Geometry: final body of the model. Coordinates: model frame, mm. Give positions to 0.01 mm unless a question says otherwise; leave off trailing zeros. Use a Markdown table: item, result. Add a question column.
1) Line query: line 1 (Z direction, x = 44, y = 15); line 2 (Z direction, x = 335.5, y = -21.5); line 3 (Z direction, x = -232.5, y = 0.5). Output: solid intervals per line, ascending.
2) Pin query (flat end, axial travel): pin 1 (1.9 mm diameter, centred on x = 117, z = -14.5, fed in from +Y). Return the tip coordinate at first contact, or that it passes through.
3) Section A-A on x = -64.5. State how many separate pieces and enclosed holes the cut face has, then the cut area to 3 significant figures.
```python
from build123d import *

# Parameters (mm, degrees)
SKETCH_14_R                 = 3
SKETCH_14_R_2               = 2.5
GB_T5237_2004_6060G_1_DEPTH = 850


with BuildPart() as part:
    # 草图14 → 铝型材（gb t5237-2004） 6060G(1) (new body)
    with BuildSketch(Plane.YZ.offset(-425)):
        with BuildLine():
            Line((28, -18.15), (30, -18.15))
            Line((30, -18.15), (30, -29.5))
            ThreePointArc((30, -29.5), (29.853553391, -29.853553391), (29.5, -30))
            Line((29.5, -30), (18.15, -30))
            Line((18.15, -30), (18.15, -28))
            Line((18.15, -28), (20.15, -28))
            Line((20.15, -28), (20.15, -22))
            Line((20.15, -22), (18.15, -22))
            Line((18.15, -22), (18.15, -20))
            Line((18.15, -20), (11.85, -20))
            Line((11.85, -20), (11.85, -22))
            Line((11.85, -22), (9.85, -22))
            Line((9.85, -22), (9.85, -28))
            Line((9.85, -28), (11.85, -28))
            Line((11.85, -28), (11.85, -30))
            Line((11.85, -30), (-11.85, -30))
            Line((-11.85, -30), (-11.85, -28))
            Line((-11.85, -28), (-9.85, -28))
            Line((-9.85, -28), (-9.85, -22))
            Line((-9.85, -22), (-11.85, -22))
            Line((-11.85, -22), (-11.85, -20))
            Line((-11.85, -20), (-18.15, -20))
            Line((-18.15, -20), (-18.15, -22))
            Line((-18.15, -22), (-20.15, -22))
            Line((-20.15, -22), (-20.15, -28))
            Line((-20.15, -28), (-18.15, -28))
            Line((-18.15, -28), (-18.15, -30))
            Line((-18.15, -30), (-29.5, -30))
            ThreePointArc((-29.5, -30), (-29.853553391, -29.853553391), (-30, -29.5))
            Line((-30, -29.5), (-30, -18.15))
            Line((-30, -18.15), (-28, -18.15))
            Line((-28, -18.15), (-28, -20.15))
            Line((-28, -20.15), (-22, -20.15))
            Line((-22, -20.15), (-22, -18.15))
            Line((-22, -18.15), (-20, -18.15))
            Line((-20, -18.15), (-20, -11.85))
            Line((-20, -11.85), (-22, -11.85))
            Line((-22, -11.85), (-22, -9.85))
            Line((-22, -9.85), (-28, -9.85))
            Line((-28, -9.85), (-28, -11.85))
            Line((-28, -11.85), (-30, -11.85))
            Line((-30, -11.85), (-30, 11.85))
            Line((-30, 11.85), (-28, 11.85))
            Line((-28, 11.85), (-28, 9.85))
            Line((-28, 9.85), (-22, 9.85))
            Line((-22, 9.85), (-22, 11.85))
            Line((-22, 11.85), (-20, 11.85))
            Line((-20, 11.85), (-20, 18.15))
            Line((-20, 18.15), (-22, 18.15))
            Line((-22, 18.15), (-22, 20.15))
            Line((-22, 20.15), (-28, 20.15))
            Line((-28, 20.15), (-28, 18.15))
            Line((-28, 18.15), (-30, 18.15))
            Line((-30, 18.15), (-30, 29.5))
            ThreePointArc((-30, 29.5), (-29.853553391, 29.853553391), (-29.5, 30))
            Line((-29.5, 30), (-18.15, 30))
            Line((-18.15, 30), (-18.15, 28))
            Line((-18.15, 28), (-20.15, 28))
            Line((-20.15, 28), (-20.15, 22))
            Line((-20.15, 22), (-18.15, 22))
            Line((-18.15, 22), (-18.15, 20))
            Line((-18.15, 20), (-11.85, 20))
            Line((-11.85, 20), (-11.85, 22))
            Line((-11.85, 22), (-9.85, 22))
            Line((-9.85, 22), (-9.85, 28))
            Line((-9.85, 28), (-11.85, 28))
            Line((-11.85, 28), (-11.85, 30))
            Line((-11.85, 30), (11.85, 30))
            Line((11.85, 30), (11.85, 28))
            Line((11.85, 28), (9.85, 28))
            Line((9.85, 28), (9.85, 22))
            Line((9.85, 22), (11.85, 22))
            Line((11.85, 22), (11.85, 20))
            Line((11.85, 20), (18.15, 20))
            Line((18.15, 20), (18.15, 22))
            Line((18.15, 22), (20.15, 22))
            Line((20.15, 22), (20.15, 28))
            Line((20.15, 28), (18.15, 28))
            Line((18.15, 28), (18.15, 30))
            Line((18.15, 30), (29.5, 30))
            ThreePointArc((29.5, 30), (29.853553391, 29.853553391), (30, 29.5))
            Line((30, 29.5), (30, 18.15))
            Line((30, 18.15), (28, 18.15))
            Line((28, 18.15), (28, 20.15))
            Line((28, 20.15), (22, 20.15))
            Line((22, 20.15), (22, 18.15))
            Line((22, 18.15), (20, 18.15))
            Line((20, 18.15), (20, 11.85))
            Line((20, 11.85), (22, 11.85))
            Line((22, 11.85), (22, 9.85))
            Line((22, 9.85), (28, 9.85))
            Line((28, 9.85), (28, 11.85))
            Line((28, 11.85), (30, 11.85))
            Line((30, 11.85), (30, -11.85))
            Line((30, -11.85), (28, -11.85))
            Line((28, -11.85), (28, -9.85))
            Line((28, -9.85), (22, -9.85))
            Line((22, -9.85), (22, -11.85))
            Line((22, -11.85), (20, -11.85))
            Line((20, -11.85), (20, -18.15))
            Line((20, -18.15), (22, -18.15))
            Line((22, -18.15), (22, -20.15))
            Line((22, -20.15), (28, -20.15))
            Line((28, -20.15), (28, -18.15))
        make_face()
        with Locations((25, 25)):
            Circle(SKETCH_14_R, mode=Mode.SUBTRACT)
        with Locations((-15, 15)):
            Circle(SKETCH_14_R_2, mode=Mode.SUBTRACT)
        with Locations((-25, -25)):
            Circle(SKETCH_14_R, mode=Mode.SUBTRACT)
        with Locations((25, -25)):
            Circle(SKETCH_14_R, mode=Mode.SUBTRACT)
        with Locations((15, -15)):
            Circle(SKETCH_14_R_2, mode=Mode.SUBTRACT)
        with Locations((-15, -15)):
            Circle(SKETCH_14_R_2, mode=Mode.SUBTRACT)
        with Locations((-25, 25)):
            Circle(SKETCH_14_R, mode=Mode.SUBTRACT)
        with Locations((15, 15)):
            Circle(SKETCH_14_R_2, mode=Mode.SUBTRACT)
        with BuildLine():
            Line((18.15, -10.5), (20.8, -7.85))
            Line((20.8, -7.85), (22.5, -7.85))
            ThreePointArc((22.5, -7.85), (25.328427125, -6.678427125), (26.5, -3.85))
            Line((26.5, -3.85), (26.5, 3.85))
            ThreePointArc((26.5, 3.85), (25.328427125, 6.678427125), (22.5, 7.85))
            Line((22.5, 7.85), (20.8, 7.85))
            Line((20.8, 7.85), (18.15, 10.5))
            Line((18.15, 10.5), (15, 10.5))
            ThreePointArc((15, 10.5), (11.818019485, 11.818019485), (10.5, 15))
            Line((10.5, 15), (10.5, 18.15))
            Line((10.5, 18.15), (7.85, 20.8))
            Line((7.85, 20.8), (7.85, 22.5))
            ThreePointArc((7.85, 22.5), (6.678427125, 25.328427125), (3.85, 26.5))
            Line((3.85, 26.5), (-3.85, 26.5))
            ThreePointArc((-3.85, 26.5), (-6.678427125, 25.328427125), (-7.85, 22.5))
            Line((-7.85, 22.5), (-7.85, 20.8))
            Line((-7.85, 20.8), (-10.5, 18.15))
            Line((-10.5, 18.15), (-10.5, 15))
            ThreePointArc((-10.5, 15), (-11.818019485, 11.818019485), (-15, 10.5))
            Line((-15, 10.5), (-18.15, 10.5))
            Line((-18.15, 10.5), (-20.8, 7.85))
            Line((-20.8, 7.85), (-22.5, 7.85))
            ThreePointArc((-22.5, 7.85), (-25.328427125, 6.678427125), (-26.5, 3.85))
            Line((-26.5, 3.85), (-26.5, -3.85))
            ThreePointArc((-26.5, -3.85), (-25.328427125, -6.678427125), (-22.5, -7.85))
            Line((-22.5, -7.85), (-20.8, -7.85))
            Line((-20.8, -7.85), (-18.15, -10.5))
            Line((-18.15, -10.5), (-15, -10.5))
            ThreePointArc((-15, -10.5), (-11.818019485, -11.818019485), (-10.5, -15))
            Line((-10.5, -15), (-10.5, -18.15))
            Line((-10.5, -18.15), (-7.85, -20.8))
            Line((-7.85, -20.8), (-7.85, -22.5))
            ThreePointArc((-7.85, -22.5), (-6.678427125, -25.328427125), (-3.85, -26.5))
            Line((-3.85, -26.5), (3.85, -26.5))
            ThreePointArc((3.85, -26.5), (6.678427125, -25.328427125), (7.85, -22.5))
            Line((7.85, -22.5), (7.85, -20.8))
            Line((7.85, -20.8), (10.5, -18.15))
            Line((10.5, -18.15), (10.5, -15))
            ThreePointArc((10.5, -15), (11.818019485, -11.818019485), (15, -10.5))
            Line((15, -10.5), (18.15, -10.5))
        make_face(mode=Mode.SUBTRACT)
    extrude(amount=GB_T5237_2004_6060G_1_DEPTH)


solid = part.part
```
Found:
| question | item | result |
|---|---|---|
| 1 | line 1 | -20 to -17.5, -12.5 to -10.5, 10.5 to 12.5, 17.5 to 20 |
| 1 | line 2 | -30 to -18.15, -11.85 to -7.85, 7.85 to 11.85, 18.15 to 30 |
| 1 | line 3 | -30 to -26.5, 26.5 to 30 |
| 2 | pin 1 | y = 20 |
| 3 | separate pieces | 1 |
| 3 | enclosed holes | 9 |
| 3 | area | 1,090 mm² |
